from build123d import *

# Parameters (mm, degrees)
F0_W     = 55
F0_H     = 55
F0_R     = 3.132813
F0_R_2   = 3.273598
F0_R_3   = 3
F0_R_4   = 3.290695
F0_R_5   = 3.156981
F1_DEPTH = 2.54
F3_DEPTH = 2.54
F4_DEPTH = 2.54


with BuildPart() as f1:
    # F0 (on Front) → F1 (new body)
    with BuildSketch(Plane.XZ):
        Rectangle(F0_W, F0_H)
        with Locations((0, -13)):
            Circle(F0_R, mode=Mode.SUBTRACT)
        with Locations((-13, 0)):
            Circle(F0_R_2, mode=Mode.SUBTRACT)
        Circle(F0_R_3, mode=Mode.SUBTRACT)
        with Locations((13, 0)):
            Circle(F0_R_4, mode=Mode.SUBTRACT)
        with Locations((0, 13)):
            Circle(F0_R_5, mode=Mode.SUBTRACT)
    extrude(amount=F1_DEPTH)

    # F2 (on Front) → F3 (join)
    with BuildSketch(Plane.XZ):
        Polygon((27.176162, 56.960059), (-2.272366, 26.004693), (-2.272366, 25.895225), (15.78599, 8.715909), (45.289185, 39.728738), align=None)
    extrude(amount=F3_DEPTH)

    # F2 (on Front) → F4 (join)
    with BuildSketch(Plane.XZ):
        Polygon((-5.332045, -25.728772), (-23.22517, -8.266557), (-53.441247, -38.482634), (-35.763578, -56.160304), align=None)
        Polygon((19.693311, -8.566808), (2.620379, -26.830509), (31.317548, -54.130764), (48.548869, -36.017741), align=None)
        Polygon((-26.064494, 6.253897), (-10.96375, 26.182832), (-42.571661, 51.02363), (-58.019511, 31.367487), align=None)
    extrude(amount=F4_DEPTH)


solid = f1.part
Check sheet for the modelled part. Datum: model origin and axes. Units: mm. A direction names the side the tool comes from. Give positions to 0.01 mm unless a question says otherwise; leave off trailing zeros. Loops run counter-clockwise (first coordinate to the right, second up) from the corner with the lowest first, then second, coordinate; pieces in that order, holes last. Notation, with made-up numbers: M 28,42.5 L 54,42.5 A24 cw 54,57.5 Z; hole C 60,-19.5 d4. An arc over 180 degrees is marked long. Return JSON: item names as keys, results as strings. Group by question number.
1. Cross-section at A-A on y = -1.55. Record the boundary of the cut face in (x, z), plus the area to 3 significant figures.
2. Cross-section at B-B on z = 0. Record the boundary of the cut face in (x, y).
3. Mould release check, pull along Z, two halves, no side actions. Record for faces 1 (the flat face through (-7, -1, 27.5)), 2 (the flat face through (-5, 0, 1)), 3 (the flat face through (27.5, -1, 2)), 4 (the cylindrical face through (1.7, -1.25, 15.66)): released by +Z, released by -Z, zero draft, split by the parting line, or undercut.
4. Thickness scan on L1, parallel to Z at x = 14, y = -0.75; L2, parallel to Z at x = -13, y = -1; L3, parallel to X at y = -0.6, z = 30. Record the ranges inside material, lowest first.
5. Cross-section at D-D on z = 45. Record the boundary of the cut face in (x, y), plus the area to 3 significant figures.
6. Go/stop test with flat-tipped pins: pin 1 (6 mm diameter, centred on x = -13, z = 0, fed in from +Y); pin 2 (1.3 mm diameter, centred on x = -3, y = -1, fed in from -Z). Record where each tip stops, or that it passes through.
7. Cross-section at C-C on x = 34. Record the boundary of the cut face in (y, z), plus the area to 3 significant figures.
8. Tool access check on faces 5 (the flat face through (13.359, -1.252, 42.436)), 6 (the flat face through (17.125, -1.252, -40.629)), 7 (the flat face through (-42.97, -1.25, 19.54)), 8 (the flat face through (36.27, -1.25, 30.25)). Record the directions out of +Z, -Z, +X, -X, +Y, -Y that give a thin tool (end or side, any length) a straight path to the whole face; none if there is none.
Return value:
{
 "1": {"outline": "M -58.02,31.37 L -27.5,7.38 L -27.5,-12.54 L -53.44,-38.48 L -35.76,-56.16 L -7.1,-27.5 L 3.32,-27.5 L 31.32,-54.13 L 48.55,-36.02 L 27.5,-15.99 L 27.5,21.03 L 45.29,39.73 L 27.18,56.96 L -0.85,27.5 L -12.64,27.5 L -42.57,51.02 Z; hole C -13,0 d6.55; hole C 0,13 d6.31; hole C 0,-13 d6.27; hole C 0,0 d6; hole C 13,0 d6.58", "area": "5,940 mm^2"},
 "2": {"outline": "M -27.5,-2.54 L -16.27,-2.54 L -16.27,0 L -27.5,0 Z; M -9.73,-2.54 L -3,-2.54 L -3,0 L -9.73,0 Z; M 3,-2.54 L 9.71,-2.54 L 9.71,0 L 3,0 Z; M 16.29,-2.54 L 27.5,-2.54 L 27.5,0 L 16.29,0 Z"},
 "3": {"face 1": "released by +Z", "face 2": "zero draft", "face 3": "undercut", "face 4": "undercut"},
 "4": {"L1": "-37.66 to -3.14, 3.14 to 43.11", "L2": "-33.4 to -3.27, 3.27 to 27.78", "L3": "-56.28 to -15.82, 1.53 to 36.03"},
 "5": {"outline": "M -47.31,-2.54 L -34.91,-2.54 L -34.91,0 L -47.31,0 Z; M 15.8,-2.54 L 39.75,-2.54 L 39.75,0 L 15.8,0 Z", "area": "92.3 mm^2"},
 "6": {"pin 1": "through", "pin 2": "z = -27.5"},
 "7": {"outline": "M -2.54,-51.31 L 0,-51.31 L 0,-22.18 L -2.54,-22.18 Z; M -2.54,27.86 L 0,27.86 L 0,50.47 L -2.54,50.47 Z", "area": "131 mm^2"},
 "8": {"face 5": "+Z, +Y, -Y", "face 6": "-Z, +Y, -Y", "face 7": "-X, +Y, -Y", "face 8": "+X, +Y, -Y"}
}
